Work out the finished part from the listing and answer in its coordinate system (mm). A direction names the side the tool comes from. Round coordinates to 2 decimals unless told otherwise and drop trailing zeros. Write each loop counter-clockwise with the first axis right and the second up, starting at its lowest first coordinate (ties: lowest second). Pieces come first, ordered by that corner, then holes. Notation, with made-up numbers: M 63,-27 L 103,-27 A20 ccw 103,6 Z; hole C 53.25,77.5 d10. An arc over 180 degrees is marked long. One line per item, written item: value. Start each with the question number.
Q1. Given pin 1 Ø1.8 at (x, y) = (76.5, 7.5) entering from +Z; pin 2 Ø1.8 at (x, y) = (33.5, 6.5) entering from -Z, each flat-ended and moving along its own axis, determine where each tip first touches the part or whether it passes through.
Q2. Find section C-C (y = 7.5). Count the separate pieces of the cut face and the enclosed holes in it, and give its area (3 significant figures).
Q3. Find section A-A (z = -39.5). Write down the section's boundary in (x, y).
Q4. Consider probe 1 along X at (y, z) = (4.75, 18.5); probe 2 along Z at (x, y) = (-88, 12.25); probe 3 along X at (y, z) = (5.5, -44). Determine where each line is inside the solid, lowest interval first.
Q5. A tool of negligible diameter and unlimited length cuts with its end or side. For faces 1 (the flat face through (-7, 7, 33.207)), 2 (the flat face through (-82.5, 9.1, 22.275)), 3 (the flat face through (94.869, 7, -11)), 4 (the cylindrical face through (-42.134, 7.632, -39.362)), 5 (the cylindrical face through (-88.442, 7.632, 15.777)), from which of +Z, -Z, +X, -X, +Y, -Y can it reach the whole face along a straight path? Write none if from no direction.
Q6. The mould has two halves that part along Y. Classify faces 6 (the cylindrical face through (77.249, 5.675, -51.403)), 7 (the cylindrical face through (-88.442, 7.632, 27.818)), 8 (the flat face through (30.869, 7, -44)), 9 (the flat face through (-7, 0, -12)): released by +Y, released by -Y, zero draft, split by the parting line, or undercut.
Q7. Find section B-B (z = -22.5). Write down the section's boundary in (x, y), and give its area (3 significant figures).
from build123d import *

# Parameters (mm, degrees)
SKETCH1_W           = 200
SKETCH1_H           = 90
SKETCH1_R           = 3
SKETCH1_W_2         = 8
SKETCH1_H_2         = 4
BOSS_EXTRUDE1_DEPTH = 15
SKETCH2_R           = 3
CUT_EXTRUDE1_DEPTH  = 20
SKETCH3_R           = 3
CUT_EXTRUDE2_DEPTH  = 20


with BuildPart() as part:
    # Sketch1 → Boss-Extrude1 (new body)
    with BuildSketch(Plane(origin=(0, 0, 0), x_dir=(1, 0, 0), z_dir=(0, 1, 0))):
        with Locations((-5.131403118, 11.792873051)):
            Rectangle(SKETCH1_W, SKETCH1_H)
        with Locations(Location((-15.131403118, 21.792873051, 0), (0, 0, 270))):
            Circle(SKETCH1_R, mode=Mode.SUBTRACT)
        with Locations(Location((-15.131403118, 1.792873051, 0), (0, 0, 90))):
            Circle(SKETCH1_R, mode=Mode.SUBTRACT)
        with Locations(Location((4.868596882, 21.792873051, 0), (0, 0, 90))):
            Circle(SKETCH1_R, mode=Mode.SUBTRACT)
        with Locations(Location((4.868596882, 1.792873051, 0), (0, 0, 270))):
            Circle(SKETCH1_R, mode=Mode.SUBTRACT)
        with Locations(Location((84.868596882, -13.207126949, 0), (0, 0, 270))):
            Circle(SKETCH1_R, mode=Mode.SUBTRACT)
        with Locations((-85.131403118, 43.860843617)):
            Rectangle(SKETCH1_W_2, SKETCH1_H_2, mode=Mode.SUBTRACT)
        with Locations((-45.131403118, 43.860843617)):
            Rectangle(SKETCH1_W_2, SKETCH1_H_2, mode=Mode.SUBTRACT)
        with Locations((34.868596882, 43.860843617)):
            Rectangle(SKETCH1_W_2, SKETCH1_H_2, mode=Mode.SUBTRACT)
        with Locations((74.868596882, 43.860843617)):
            Rectangle(SKETCH1_W_2, SKETCH1_H_2, mode=Mode.SUBTRACT)
        with Locations((74.868596882, -20.275097514)):
            Rectangle(SKETCH1_W_2, SKETCH1_H_2, mode=Mode.SUBTRACT)
        with Locations((-85.131403118, -20.275097514)):
            Rectangle(SKETCH1_W_2, SKETCH1_H_2, mode=Mode.SUBTRACT)
    extrude(amount=BOSS_EXTRUDE1_DEPTH)

    # Sketch2 → Cut-Extrude1 (cut)
    with BuildSketch(Plane(origin=(0, 0, -56.792873051), x_dir=(-1, 0, 0), z_dir=(0, 0, -1))):
        with Locations((-74.868596882, 7.5)):
            Circle(SKETCH2_R)
        with Locations((-34.868596882, 7.5)):
            Circle(SKETCH2_R)
        with Locations((45.131403118, 7.5)):
            Circle(SKETCH2_R)
        with Locations(Location((85.131403118, 7.5, 0), (0, 0, 180))):
            Circle(SKETCH2_R)
    extrude(amount=-CUT_EXTRUDE1_DEPTH, mode=Mode.SUBTRACT)

    # Sketch3 → Cut-Extrude2 (cut)
    with BuildSketch(Plane.XY.offset(33.207126949)):
        with Locations((-85.445029849, 7.5)):
            Circle(SKETCH3_R)
        with Locations((75.182223613, 7.5)):
            Circle(SKETCH3_R)
    extrude(amount=-CUT_EXTRUDE2_DEPTH, mode=Mode.SUBTRACT)


solid = part.part
The answers:
1. pin 1: z = 13.21
1. pin 2: z = -36.79
2. separate pieces: 1
2. enclosed holes: 5
2. area: 17,100 mm2
3. outline: M -105.13,0 L 94.87,0 L 94.87,15 L -105.13,15 Z; hole C -85.13,7.5 d6; hole C -45.13,7.5 d6; hole C 34.87,7.5 d6; hole C 74.87,7.5 d6
4. probe 1: -105.13 to -89.13, -81.13 to 70.87, 78.87 to 94.87
4. probe 2: -56.79 to -45.86, -41.86 to 18.28, 22.28 to 33.21
4. probe 3: -105.13 to -89.13, -81.13 to -49.13, -41.13 to 30.87, 38.87 to 70.87, 78.87 to 94.87
5. face 1: +Z, +X, -X, +Y, -Y
5. face 2: +Y, -Y
5. face 3: +Z, -Z, +X, +Y, -Y
5. face 4: -Z
5. face 5: +Z
6. face 6: undercut
6. face 7: undercut
6. face 8: zero draft
6. face 9: released by -Y
7. outline: M -105.13,0 L -18.05,0 L -18.05,15 L -105.13,15 Z; M -12.22,0 L 1.95,0 L 1.95,15 L -12.22,15 Z; M 7.78,0 L 94.87,0 L 94.87,15 L 7.78,15 Z
7. area: 2,830 mm2
